Autodesk Inventor part; units mm, degrees
ref_plane "YZ Plane" through (0, 0, 0) normal (1, 0, 0) x (0, 1, 0)
ref_plane "XZ Plane" through (0, 0, 0) normal (0, 1, 0) x (-1, 0, 0)
ref_plane "XY Plane" through (0, 0, 0) normal (0, 0, 1) x (1, 0, 0)
sketch "Sketch1" plane through (0, 0, 0) normal (1, 0, 0) x (0, 1, 0)
  line L0 (20, 0) -> (20, 3)
  line L1 (20, 3) -> (4, 3)
  line L2 (4, 3) -> (4, 34)
  line L3 (4, 34) -> (0, 34)
  line L4 (0, 34) -> (0, 0)
  line L5 (0, 0) -> (20, 0)
  dimension "d0" = 3
  dimension "d1" = 4
  dimension "d2" = 34
  dimension "d3" = 20
extrude "Extrusion1" add sketch "Sketch1" along normal blind 26
sketch "Sketch2" plane through (0, 4, 34) normal (0, 1, 0) x (1, 0, 0)
  line L0 (0, 31) -> (0, 0)
  line L1 (0, 0) -> (26, 0)
  line L2 (0, 31) -> (26, 31)
  point P0 (0, 34)
  point P1 (13, 7)
  point P2 (13, 24)
  dimension "d6" = 7
  dimension "d8" = 13
  dimension "d16" = 26
  dimension "d17" = 31
  dimension "d19" = 7
hole "Hole1" at (13, 4, 27) at (13, 4, 10) direction (0, -1, 0) diameter 2.459 end through all counterbore diameter 6 counterbore depth 3
sketch "Sketch3" plane through (0, 4, 3) normal (0, 0, 1) x (1, 0, 0)
  line L0 (0, 16) -> (0, 0)
  line L1 (0, 16) -> (26, 16)
  circle A0 centre (13, 13) radius 1.05
  line L2 (11.95, 13) -> (11.95, 16)
  line L3 (14.05, 13) -> (14.05, 16)
  point P0 (0, -4)
  dimension "d20" = 2.1
  dimension "d21" = 13
  dimension "d22" = 3
  dimension "d28" = 26
extrude "Extrusion2" cut sketch "Sketch3" against normal through all
sketch "Sketch4" plane through (0, 4, 3) normal (0, 0, 1) x (1, 0, 0)
  arc A0 (11.95, 13) -> (14.05, 13) centre (13, 13) ccw
  circle A1 centre (13, 13) radius 2.1
  line L0 (0, 16) -> (11.95, 16)
  line L1 (14.05, 16) -> (26, 16)
  line L2 (10.9, 13) -> (10.9, 16)
  line L3 (15.1, 13) -> (15.1, 16)
  line L4 (10.9, 16) -> (15.1, 16)
  point P0 (0, -4)
  dimension "d25" = 4.2
extrude "Extrusion3" cut sketch "Sketch4" against normal blind 0.5
equation "\"d21\" = 0.5 * d28"
properties part number "SupportSlide" material "Aluminum"
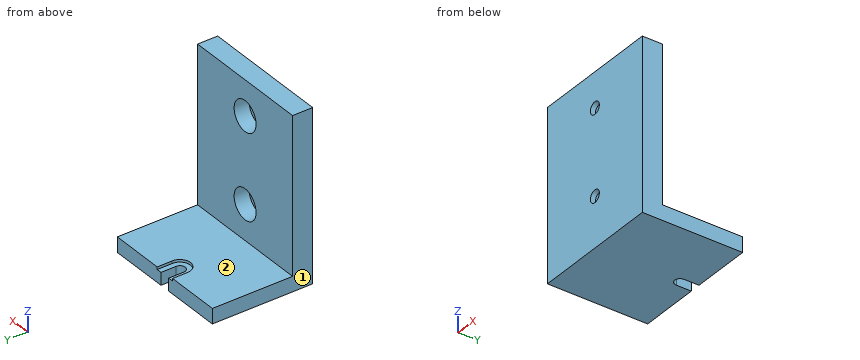
Work out the finished part from the listing and answer in its coordinate system (mm). Face numbers are marked on the shaded views. A direction names the side the tool comes from. Give positions to 0.01 mm unless a question says otherwise; leave off trailing zeros. Loops run counter-clockwise (first coordinate to the right, second up) from the corner with the lowest first, then second, coordinate; pieces in that order, holes last. Notation, with made-up numbers: (-4.75, -18) -> (28.25, -18) arc R23 cw to (28.25, -5) -> close; hole circle Ø7 at (88.25, 67). An arc over 180 degrees is marked (long way). Write item = value, one per line. Start each with the question number.
(1) Find section A-A on z = 27. Give the vertices of the cut face in (x, y), and give its area (3 significant figures).
(2) Find section C-C on y = 8.75. Give the vertices of the cut face in (x, z), and give its area (3 significant figures).
(3) Find the intervals of material crossed by probe 1 along Z at (x, y) = (13, 0.75); probe 2 along Z at (x, y) = (13, 2.8); probe 3 along X at (y, z) = (2.6, 27), in increasing order. Write a range as from..to.
(4) Given pin 1 Ø13 at (x, z) = (18.5, 20) entering from +Y; pin 2 Ø2 at (x, y) = (13.5, 18.5) entering from +Z; pin 3 Ø5.5 at (x, z) = (13, 27) entering from +Y, each flat-ended and moving along its own axis, determine where each tip first touches the part or whether it passes through.
(5) Find section B-B on x = 5.75. Give the vertices of the cut face in (y, z).
(6) Find section D-D on z = 17.5. Give the vertices of the cut face in (x, y).
(7) Which of the six approach directions +Z, -Z, +X, -X, +Y, -Y give full straight-line access (tool end or side, diameter ignored) to the marked faces 1 and 2?
From the geometry:
q1.outline = (0, 0) -> (11.77, 0) -> (11.77, 1) -> (10, 1) -> (10, 4) -> (0, 4) -> close; (14.23, 0) -> (26, 0) -> (26, 4) -> (16, 4) -> (16, 1) -> (14.23, 1) -> close
q1.area = 83.5 mm^2
q2.outline = (0, 0) -> (26, 0) -> (26, 3) -> (0, 3) -> close
q2.area = 78.0 mm^2
q3.probe_1 = 0..8.77, 11.23..25.77, 28.23..34
q3.probe_2 = 0..7, 13..24, 30..34
q3.probe_3 = 0..10, 16..26
q4.pin_1 = 4
q4.pin_2 = 2.5
q4.pin_3 = 1
q5.outline = (0, 0) -> (20, 0) -> (20, 3) -> (4, 3) -> (4, 34) -> (0, 34) -> close
q6.outline = (0, 0) -> (26, 0) -> (26, 4) -> (0, 4) -> close
q7.face_1 = +Z, -Z, -X, +Y, -Y
q7.face_2 = +Z, +X, -X, +Y
